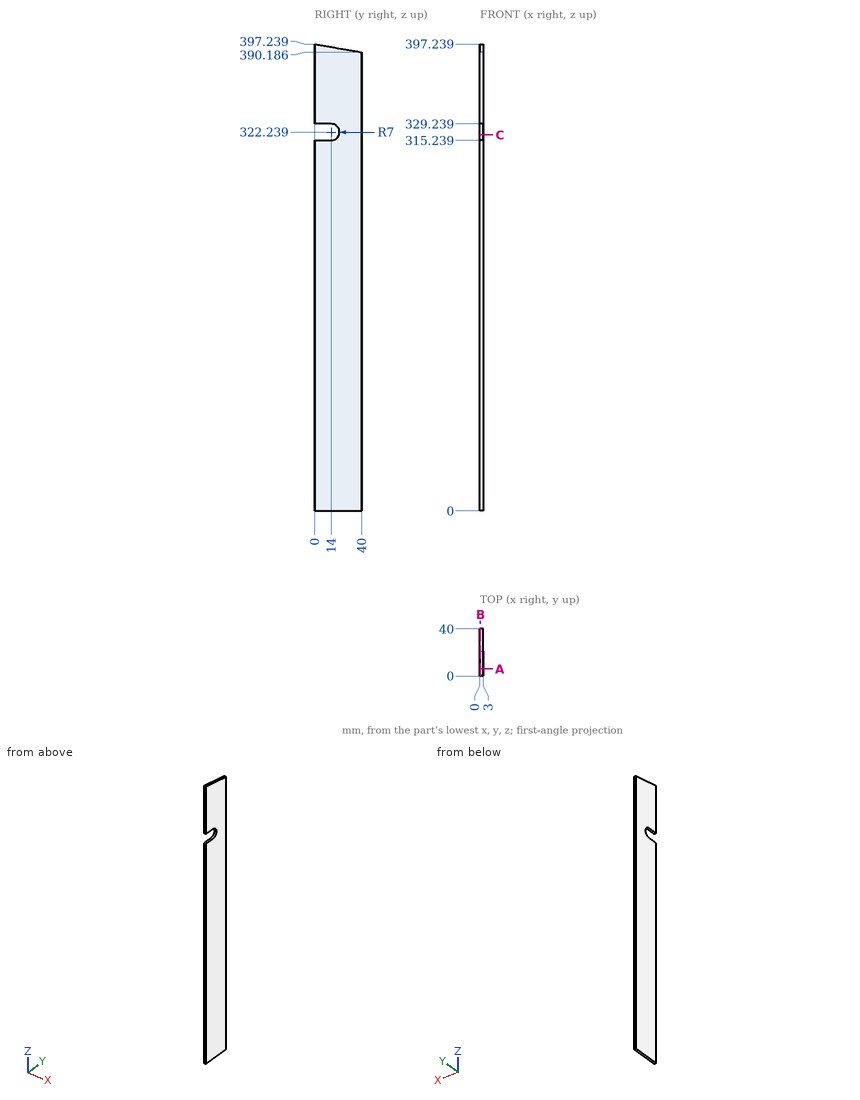
The figure shows three views and two pictorial views of one solid part (mm, origin at its lowest corner). Answer the questions. Give positions to 0.01 mm unless a question says otherwise; leave off trailing zeros. Order: outer loops, then holes, each group sorted by start corner. A loop starts at its lowest first (then second) coordinate and runs counter-clockwise, first axis right, second up. Notation, with made-up numbers: (44, -6.75) -> (103, -6.75) arc R33 cw to (103, 21.25) -> close; hole circle Ø6 at (54.25, 89). An arc over 180 degrees is marked (long way). Answer as a JSON object with one key per item and string values. Group by question number.
Item 1: The part is cut by section B-B on x = 0.6. Write down the section's boundary in (y, z), and give its area (3 significant figures).
Item 2: The part is cut by section A-A on y = 6. Write down the section's boundary in (x, z).
Item 3: A flat-ended cylindrical pin translates along its axis: pin 1 (1.5 mm diameter, centred on x = 1, y = 5.5, fed in from +Z). Find the tip coordinate at first contact, or state that the pin passes through.
Item 4: Consider L1, parallel to Z at x = 2.25, y = 8; L2, parallel to Z at x = 2.2, y = 4; L3, parallel to Z at x = 2.5, y = 28.5. Determine where each line is inside the solid, lowest interval first. Write a range as from..to.
Item 5: The part is cut by section C-C on z = 320. Write down the section's boundary in (x, y), and give its area (3 significant figures).
Result set:
{
 "1": {"outline": "(0, 0) -> (40, 0) -> (40, 390.19) -> (0, 397.24) -> (0, 329.24) -> (14, 329.24) arc R7 cw to (14, 315.24) -> (0, 315.24) -> close", "area": "15,500 mm²"},
 "2": {"outline": "(0, 0) -> (3, 0) -> (3, 315.24) -> (0, 315.24) -> close; (0, 329.24) -> (3, 329.24) -> (3, 396.18) -> (0, 396.18) -> close"},
 "3": {"pin 1": "z = 396.4"},
 "4": {"L1": "0..315.24, 329.24..395.83", "L2": "0..315.24, 329.24..396.53", "L3": "0..392.21"},
 "5": {"outline": "(0, 20.63) -> (3, 20.63) -> (3, 40) -> (0, 40) -> close", "area": "58.1 mm²"}
}
